Answer from the drawing. Dimensions are ordinates in mm from the lowest x, y and z of the part. Coordinates: 2 decimals unless noted, no trailing zeros. Loops run counter-clockwise (first coordinate to the right, second up) from the corner with the lowest first, then second, coordinate; pieces in that order, holes last. Notation, with made-up numbers: M -15,10 L 7,10 A9 cw 7,18 Z; hole C 88,68 d10. An arc over 180 degrees is marked long. Put each result on its own line as item: value.
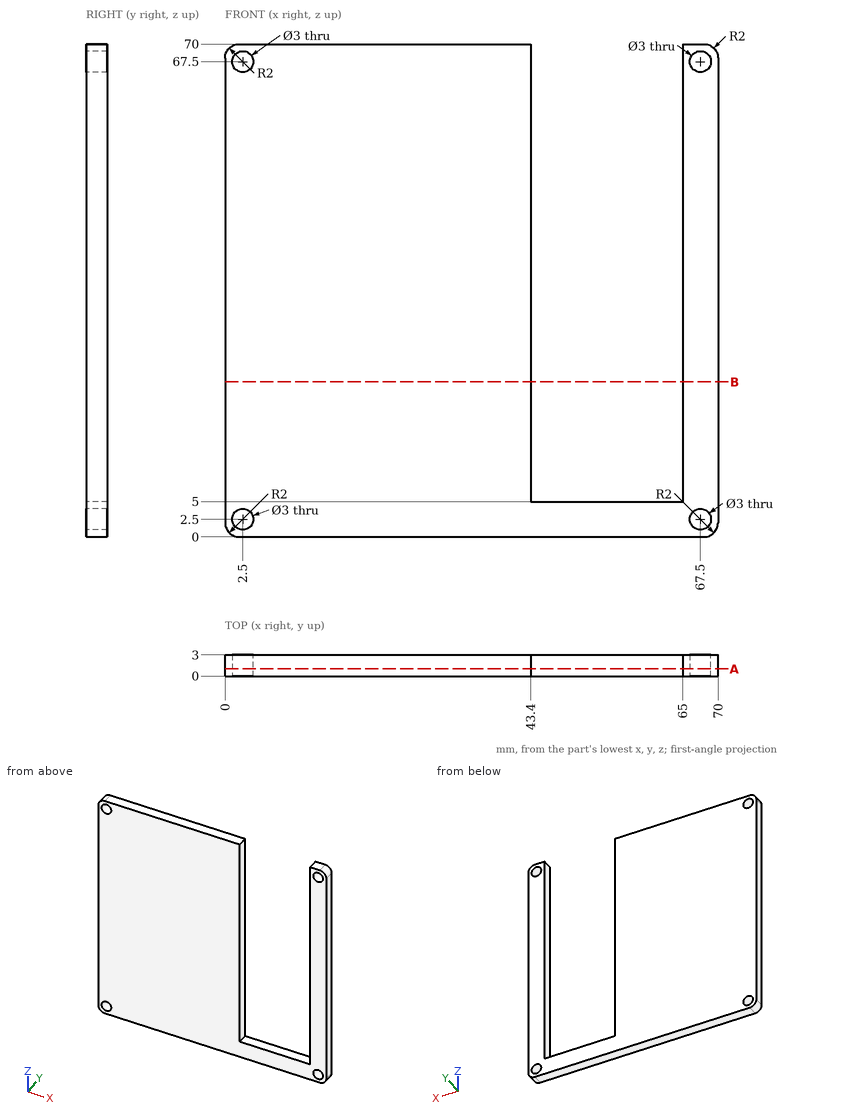
1) Find section B-B, the plane z = 22. Write down the section's boundary in (x, y), plus the area to 3 significant figures.
Answer list:
outline: M 0,0 L 43.4,0 L 43.4,3 L 0,3 Z; M 65,0 L 70,0 L 70,3 L 65,3 Z
area: 145 mm^2
2) Given pin 1 Ø4 at (x, z) = (2.5, 67.5) entering from -Y; pin 2 Ø1 at (x, y) = (48.5, 1.5) entering from +Z, each flat-ended and moving along its own axis, determine where each tip first touches the part or whether it passes through.
Answer list:
pin 1: stops at y = 0
pin 2: stops at z = 5
3) Find section A-A, the plane y = 1. Write down the section's boundary in (x, z).
Answer list:
outline: M 0,2 A2 ccw 2,0 L 68,0 A2 ccw 70,2 L 70,68 A2 ccw 68,70 L 65,70 L 65,5 L 43.4,5 L 43.4,70 L 2,70 A2 ccw 0,68 Z; hole C 2.5,2.5 d3; hole C 2.5,67.5 d3; hole C 67.5,2.5 d3; hole C 67.5,67.5 d3
4) Straight lines are drawn through the part: line 1 (Z direction, x = 2.5, y = 2.45); line 2 (X direction, y = 2.1, z = 47.5). For each, find the intervals that lie inside material, in ascending order. Write a range as [from, to].
Answer list:
line 1: z = [0, 1], [4, 66], [69, 70]
line 2: x = [0, 43.4], [65, 70]
